Could you check a few things on this drawing? It's one solid part, dimensions in mm from its lowest x, y, z. A direction names the side the tool comes from. Round coordinates to 2 decimals unless told otherwise and drop trailing zeros. Order: outer loops, then holes, each group sorted by start corner. A loop starts at its lowest first (then second) coordinate and runs counter-clockwise, first axis right, second up.
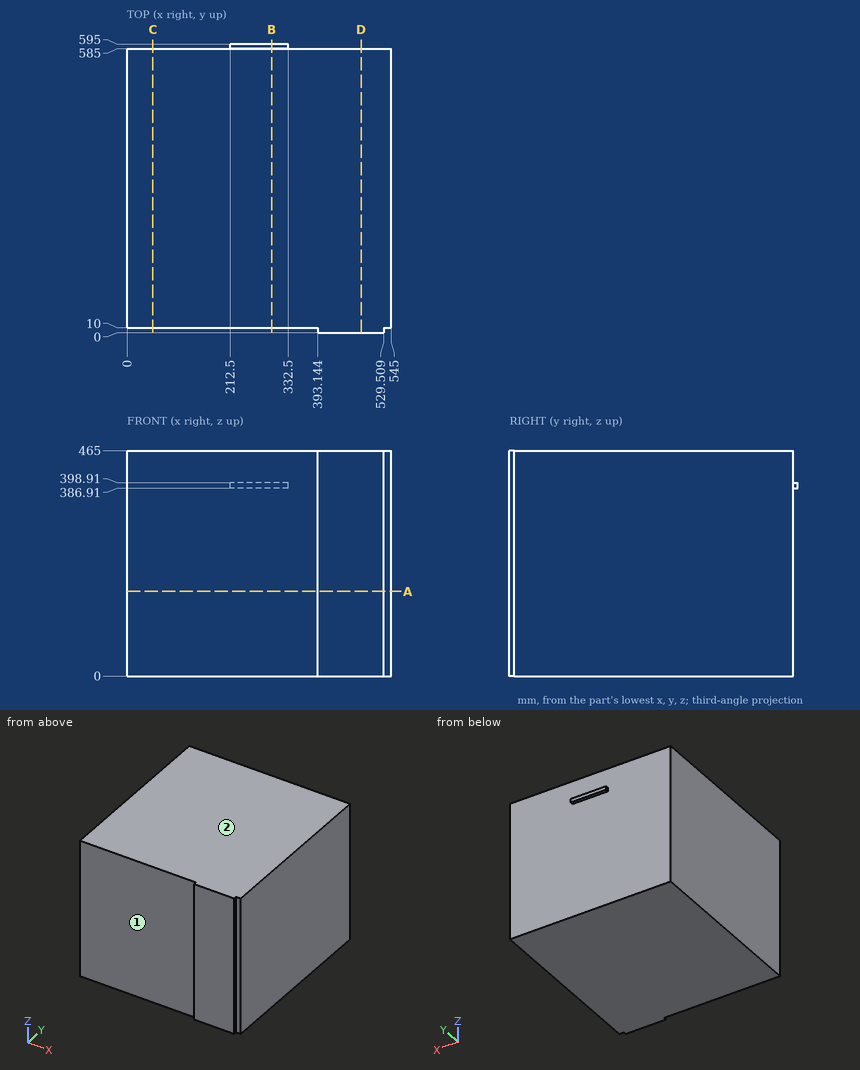
1) If we section it at A-A (z = 174.5): Write out the boundary of the cut face in (x, y).
2) I need wall thicknesses on line 1 (Y direction, x = 134, z = 88.5); line 2 (Y direction, x = 429.5, z = 251). Which ranges of each line are inside material? Lowest first, please.
3) If we section it at D-D (x = 482.5): Write out the boundary of the cut face in (y, z).
4) If we section it at B-B (x = 298): Write out the boundary of the cut face in (y, z).
5) For the marked faces 1 and 2, which set-ups out of +Z, -Z, +X, -X, +Y, -Y let a thin tool reach every point of the face, with its end or its side?
6) If we section it at C-C (x = 53): Write out the boundary of the cut face in (y, z), plus the area to 3 significant figures.
7) I'm going to push flat-ended pins straight in: pin 1 (10 mm diameter, centred on x = 341, z = 172.5, fed in from -Y); pin 2 (12 mm diameter, centred on x = 69, z = 204, fed in from +Y); pin 3 (11 mm diameter, centred on y = 2.5, z = 246.5, fed in from -X). Where does each tip first touch, or does it pass through?
Solutions:
1. outline: (0, 10) - (393.14, 10) - (393.14, 0) - (529.51, 0) - (529.51, 10) - (545, 10) - (545, 585) - (0, 585) - close
2. line 1: y = 10 to 585
2. line 2: y = 0 to 585
3. outline: (0, 0) - (585, 0) - (585, 465) - (0, 465) - close
4. outline: (10, 0) - (585, 0) - (585, 386.91) - (595, 386.91) - (595, 398.91) - (585, 398.91) - (585, 465) - (10, 465) - close
5. face 1: +Z, -Z, -X, -Y
5. face 2: +Z, +X, -X, +Y, -Y
6. outline: (10, 0) - (585, 0) - (585, 465) - (10, 465) - close
6. area: 267,000 mm2
7. pin 1: stops at y = 10
7. pin 2: stops at y = 585
7. pin 3: stops at x = 393.14
